CAD build for the part. Positions are in the model's coordinates, mm. A direction names the side the tool comes from. Coordinates: 2 decimals unless noted, no trailing zeros. Order: outer loops, then holes, each group sorted by start corner. A loop starts at its lowest first (then second) coordinate and runs counter-clockwise, first axis right, second up. Notation, with made-up numbers: M 76.25,42 L 88.25,42 A19 cw 88.25,70 Z; hole C 40.5,24 d6. An arc over 180 degrees is marked long. One line per item, written item: value.
from build123d import *

# Parameters (mm, degrees)
BOSS_EXTRUDE1_DEPTH = 2.6
CUT_EXTRUDE1_DEPTH  = 0.9
SKETCH4_R           = 4.5
CUT_EXTRUDE2_DEPTH  = 16
CUT_EXTRUDE2_DRAFT  = -3
SKETCH5_R           = 3.1
CUT_EXTRUDE3_DEPTH  = 1.75
CUT_EXTRUDE4_DEPTH  = 43.200740515
CUT_EXTRUDE5_DEPTH  = 7.5
CHAMFER1_SIZE       = 1
CHAMFER1_SIZE2      = 1.056754503


with BuildPart() as part:
    # Sketch1 → Revolve1 (revolve)
    with BuildSketch(Plane(origin=(0, 0, 0), x_dir=(0, 0, -1), z_dir=(1, 0, 0)), mode=Mode.PRIVATE) as revolve1_sk:
        Polygon((34, 0), (34, 6.8), (11, 6.95), (11, 7.1), (0, 7.4), (0, 0), align=None)
    revolve(revolve1_sk.sketch.rotate(Axis((0, 0, 0), (0, 0, -1)), 90), axis=Axis((0, 0, 0), (0, 0, -1)))

    # Sketch2 → Boss-Extrude1 (add)
    with BuildSketch(Plane.XY):
        with BuildLine():
            Line((-9.832020922, 2.897216699), (-5.75, 16.75))
            Line((-5.75, 16.75), (-3.15, 16.75))
            Line((-3.15, 16.75), (-3.15, 12.55))
            Line((-3.15, 12.55), (3.15, 12.55))
            Line((3.15, 12.55), (3.15, 16.75))
            Line((3.15, 16.75), (5.75, 16.75))
            Line((5.75, 16.75), (9.832020922, 2.897216699))
            ThreePointArc((9.832020922, 2.897216699), (0, -10.25), (-9.832020922, 2.897216699))
        make_face()
    extrude(amount=-BOSS_EXTRUDE1_DEPTH)

    # Sketch3 → Cut-Extrude1 (cut)
    with BuildSketch(Plane(origin=(0, 0, -2.6), x_dir=(-1, 0, 0), z_dir=(0, 0, -1))):
        with BuildLine():
            Line((-5.821011016, 11.555986793), (-5.519758848, 6.917713659))
            ThreePointArc((-5.519758848, 6.917713659), (0, 8.85), (5.519758848, 6.917713659))
            Line((5.519758848, 6.917713659), (5.821011016, 11.555986793))
            ThreePointArc((5.821011016, 11.555986793), (0, 12.939281278), (-5.821011016, 11.555986793))
        make_face()
    extrude(amount=-CUT_EXTRUDE1_DEPTH, mode=Mode.SUBTRACT)


with BuildPart() as cut_extrude2_tool:
    # Sketch4 → Cut-Extrude2 (with draft: the straight prism first)
    with BuildSketch(Plane.XY):
        Circle(SKETCH4_R)
    extrude(amount=-CUT_EXTRUDE2_DEPTH)
    # Cut-Extrude2: the draft: its side faces are tilted about the plane it starts from
    cut_extrude2_sides = [cut_extrude2_tool.faces().sort_by_distance(p)[0] for p in [
        (-4.5, 0, -8),
    ]]
    draft(cut_extrude2_sides, Plane.XY, CUT_EXTRUDE2_DRAFT)


with BuildPart() as part_1:
    add(part.part)

    # Cut-Extrude2: cut by cut_extrude2_tool
    add(cut_extrude2_tool.part, mode=Mode.SUBTRACT)

    # Sketch5 → Cut-Extrude3 (cut)
    with BuildSketch(Plane(origin=(0, 0, -34), x_dir=(-1, 0, 0), z_dir=(0, 0, -1))):
        Circle(SKETCH5_R)
    extrude(amount=-CUT_EXTRUDE3_DEPTH, mode=Mode.SUBTRACT)

    # Sketch6 → Cut-Extrude4 (cut, through all)
    with BuildSketch(Plane(origin=(0, 12.55, 0), x_dir=(1, 0, 0), z_dir=(0, 1, 0))):
        with BuildLine():
            Line((-3.65, 20.372845894), (-3.65, 24.727154106))
            ThreePointArc((-3.65, 24.727154106), (0, 26.8), (3.65, 24.727154106))
            Line((3.65, 24.727154106), (3.65, 20.372845894))
            ThreePointArc((3.65, 20.372845894), (0, 18.3), (-3.65, 20.372845894))
        make_face()
    extrude(amount=-CUT_EXTRUDE4_DEPTH, mode=Mode.SUBTRACT)

    # Sketch7 → Cut-Extrude5 (cut)
    with BuildSketch(Plane(origin=(0, 12.55, 0), x_dir=(1, 0, 0), z_dir=(0, 1, 0))):
        with BuildLine():
            Line((4.65, 20.112788479), (4.65, 24.987211521))
            ThreePointArc((4.65, 24.987211521), (0, 27.8), (-4.65, 24.987211521))
            Line((-4.65, 24.987211521), (-4.65, 20.112788479))
            ThreePointArc((-4.65, 20.112788479), (0, 17.3), (4.65, 20.112788479))
        make_face()
    extrude(amount=-CUT_EXTRUDE5_DEPTH, mode=Mode.SUBTRACT)

    # Chamfer1
    chamfer1_edges = [part_1.edges().sort_by_distance(p)[0] for p in [
        (-4.5, 0, 0),
    ]]
    chamfer1_side = [part_1.faces().sort_by_distance(p)[0] for p in [
        (-7.465828695, 9.727786539, 0),
    ]]
    chamfer(chamfer1_edges, length=CHAMFER1_SIZE, length2=CHAMFER1_SIZE2, reference=chamfer1_side[0])


solid = part_1.part
Q1. Slice it at C-C (z = -14.5). List the corners of the cut face in (x, y).
Recorded:
outline: C 0,0 d13.85; hole C 0,0 d7.48
Q2. Which spindle directions (+Z, -Z, +X, -X, +Y, -Y) get a long thin tool onto all of the face, cutting with end or side? Do faces 5 (the face through (-4.055, 0.178, -8.423)), 6 (the face through (0.1, -0.8, -18.3)), 7 (the face through (3.33, 6.4, -6.74)), 8 (the face through (-0.1, 5.8, -17.3)), 9 (the face through (-3.15, 15, -1)). Say none if no direction does.
Recorded:
face 5: +Z
face 6: +Y, -Y
face 7: -Z
face 8: +Y
face 9: +Z, -Z, +Y
Q3. Slice it at D-D (z = -9.5). List the corners of the cut face in (x, y), plus the area to 3 significant figures.
Recorded:
outline: C 0,0 d14.28; hole C 0,0 d8
area: 110 mm^2
Q4. Mould opens along X. For faces 1 (the face through (7.762, 9.921, -1.282)), 2 (the face through (-4.53, 12.12, -2.16)), 3 (the face through (4, 16.75, -1)), 4 (the face through (0, 0, -32.25)) say: released by +X, released by -X, zero draft, split by the parting line, or undercut.
Recorded:
face 1: released by +X
face 2: undercut
face 3: zero draft
face 4: undercut
Q5. Pin check, flat tips, straight feed: pin 1 Ø0.8 at (y, z) = (15.5, -2) entering from +X; pin 2 Ø2 at (y, z) = (0.5, -21.5) entering from +X; pin 3 Ø3 at (y, z) = (-6.5, -20) entering from +X. Stop position of each tip, or through.
Recorded:
pin 1: stops at x = 6.24
pin 2: stops at x = 6.89
pin 3: stops at x = 4.74
Q6. Drill centre lines: line 1 along Y through (x, z) = (0, -33.25); line 2 along Z through (x, y) = (8.75, -5.25); line 3 along Y through (x, z) = (-1, -12.5). Where is each one in solid material? Low to high.
Recorded:
line 1: y = -6.8 to -3.1, 3.1 to 6.8
line 2: z = -2.6 to 0
line 3: y = -6.87 to -3.71, 3.71 to 6.87
Q7. Slice it at B-B (z = -26). List the corners of the cut face in (x, y), plus the area to 3 significant figures.
Recorded:
outline: M -3.96,5.05 L -3.96,5.59 A6.85 ccw -2.48,-6.39 L -2.48,5.05 Z; M 2.48,-6.39 A6.85 ccw 3.96,5.59 L 3.96,5.05 L 2.48,5.05 Z
area: 78.1 mm^2
Q8. Slice it at A-A (y = 13.25). List the corners of the cut face in (x, z), plus the area to 3 significant figures.
Recorded:
outline: M -6.78,-2.6 L -3.15,-2.6 L -3.15,0 L -6.78,0 Z; M 3.15,-2.6 L 6.78,-2.6 L 6.78,0 L 3.15,0 Z
area: 18.9 mm^2
